Verification items for the finished model (mm, model axes). Face numbers are marked on the shaded views. A direction names the side the tool comes from. Coordinates: 2 decimals unless noted, no trailing zeros. Loops run counter-clockwise (first coordinate to the right, second up) from the corner with the lowest first, then second, coordinate; pieces in that order, holes last. Notation, with made-up numbers: (20, 76.25) -> (48, 76.25) arc R25 cw to (48, 97.25) -> close; hole circle Ø9 at (85, 81). An arc over 180 degrees is marked (long way). Answer as a JSON object with one key per item and string values. Group by question number.
Q1. Gauge pin test, flat ends, axial feed: pin 1 Ø1.6 at (y, z) = (-21, 1) entering from +X; pin 2 Ø2.5 at (y, z) = (-24.5, 1.5) entering from +X; pin 3 Ø1 at (x, z) = (13.5, 1) entering from -Y; pin 4 Ø5 at (y, z) = (10.5, -23.5) entering from +X. Record the tip position at first contact, or that the pin passes through.
Q2. Cross-section at D-D on x = 21. Record the boundary of the cut face in (y, z), and give its area (3 significant figures).
Q3. Set-up check for the marked faces 4, 5, 6 and 7: record each of +Z, -Z, +X, -X, +Y, -Y from which the full face is reachable in a straight line by a thin tool's end or side.
Q4. Cross-section at A-A on z = -20.5. Record the boundary of the cut face in (x, y), and give its area (3 significant figures).
Q5. Cross-section at C-C on y = -21. Record the boundary of the cut face in (x, z), and give its area (3 significant figures).
Q6. Cross-section at B-B on y = 16. Record the boundary of the cut face in (x, z), and give its area (3 significant figures).
Q7. Release check for a two-part mould opening along X. For the marked faces 1, 2 and 3 record: released by +X, released by -X, zero draft, split by the parting line, or undercut.
Q8. Scan lines: L1, parallel to Y at x = -41, z = -10.8; L2, parallel to X at y = 8, z = -29; L3, parallel to X at y = -16, z = 0.5. Record each from-to range of solid material in increasing order.
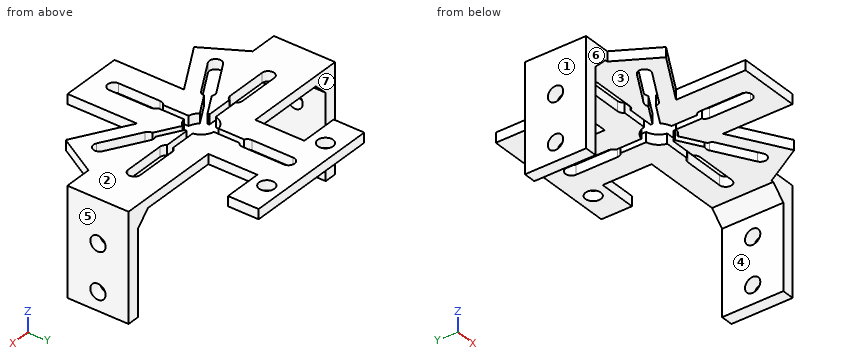
```python
from build123d import *

# Parameters (mm, degrees)
BOSS_EXTRUDE1_DEPTH = 3.2
SKETCH2_W           = 4
SKETCH2_H           = 20
BOSS_EXTRUDE2_DEPTH = 35
BOSS_EXTRUDE3_DEPTH = 20
CUT_EXTRUDE1_REACH  = 102.256
SKETCH4_R           = 2.5
SKETCH5_R           = 2.5
CUT_EXTRUDE2_DEPTH  = 3.2


with BuildPart() as part:
    # Sketch1 → Boss-Extrude1 (new body)
    with BuildSketch(Plane.XY):
        Polygon((22.5, 36), (-22.5, 36), (-22.5, 26), (-10, 26), (-10, 10), (-40, 10), (-40, -10), (-35, -10), (-27.320508076, -23.301270189), (-10, -13.301270189), (-10, -36), (10, -36), (10, -13.301270189), (27.320508076, -23.301270189), (35, -10), (40, -10), (40, 10), (10, 10), (10, 26), (22.5, 26), align=None)
        with BuildLine():
            Line((2, 28.5), (2, 15))
            ThreePointArc((2, 15), (1.732050808, 14), (1, 13.267949192))
            Line((1, 13.267949192), (1, 4.898979486))
            ThreePointArc((1, 4.898979486), (3.535533906, 3.535533906), (4.898979486, 1))
            Line((4.898979486, 1), (13.267949192, 1))
            ThreePointArc((13.267949192, 1), (14, 1.732050808), (15, 2))
            Line((15, 2), (28.5, 2))
            ThreePointArc((28.5, 2), (30.5, 0), (28.5, -2))
            Line((28.5, -2), (15, -2))
            ThreePointArc((15, -2), (14, -1.732050808), (13.267949192, -1))
            Line((13.267949192, -1), (4.898979486, -1))
            ThreePointArc((4.898979486, -1), (4.829629131, -1.294095226), (4.742640687, -1.583464339))
            Line((4.742640687, -1.583464339), (11.990381057, -5.767949192))
            ThreePointArc((11.990381057, -5.767949192), (12.990381057, -5.5), (13.990381057, -5.767949192))
            Line((13.990381057, -5.767949192), (25.681724008, -12.517949192))
            ThreePointArc((25.681724008, -12.517949192), (26.413774815, -15.25), (23.681724008, -15.982050808))
            Line((23.681724008, -15.982050808), (11.990381057, -9.232050808))
            ThreePointArc((11.990381057, -9.232050808), (11.258330249, -8.5), (10.990381057, -7.5))
            Line((10.990381057, -7.5), (3.742640687, -3.315515147))
            ThreePointArc((3.742640687, -3.315515147), (2.5, -4.330127019), (1, -4.898979486))
            Line((1, -4.898979486), (1, -13.267949192))
            ThreePointArc((1, -13.267949192), (1.732050808, -14), (2, -15))
            Line((2, -15), (2, -28.5))
            ThreePointArc((2, -28.5), (0, -30.5), (-2, -28.5))
            Line((-2, -28.5), (-2, -15))
            ThreePointArc((-2, -15), (-1.732050808, -14), (-1, -13.267949192))
            Line((-1, -13.267949192), (-1, -4.898979486))
            ThreePointArc((-1, -4.898979486), (-2.5, -4.330127019), (-3.742640687, -3.315515147))
            Line((-3.742640687, -3.315515147), (-10.990381057, -7.5))
            ThreePointArc((-10.990381057, -7.5), (-11.258330249, -8.5), (-11.990381057, -9.232050808))
            Line((-11.990381057, -9.232050808), (-23.681724008, -15.982050808))
            ThreePointArc((-23.681724008, -15.982050808), (-26.413774815, -15.25), (-25.681724008, -12.517949192))
            Line((-25.681724008, -12.517949192), (-13.990381057, -5.767949192))
            ThreePointArc((-13.990381057, -5.767949192), (-12.990381057, -5.5), (-11.990381057, -5.767949192))
            Line((-11.990381057, -5.767949192), (-4.742640687, -1.583464339))
            ThreePointArc((-4.742640687, -1.583464339), (-4.829629131, -1.294095226), (-4.898979486, -1))
            Line((-4.898979486, -1), (-13.267949192, -1))
            ThreePointArc((-13.267949192, -1), (-14, -1.732050808), (-15, -2))
            Line((-15, -2), (-28.5, -2))
            ThreePointArc((-28.5, -2), (-30.5, 0), (-28.5, 2))
            Line((-28.5, 2), (-15, 2))
            ThreePointArc((-15, 2), (-14, 1.732050808), (-13.267949192, 1))
            Line((-13.267949192, 1), (-4.898979486, 1))
            ThreePointArc((-4.898979486, 1), (-3.535533906, 3.535533906), (-1, 4.898979486))
            Line((-1, 4.898979486), (-1, 13.267949192))
            ThreePointArc((-1, 13.267949192), (-1.732050808, 14), (-2, 15))
            Line((-2, 15), (-2, 28.5))
            ThreePointArc((-2, 28.5), (0, 30.5), (2, 28.5))
        make_face(mode=Mode.SUBTRACT)
    extrude(amount=BOSS_EXTRUDE1_DEPTH)

    # Sketch2 → Boss-Extrude2 (add)
    with BuildSketch(Plane(origin=(0, 0, 3.2), x_dir=(-1, 0, 0), z_dir=(0, 0, -1))):
        with Locations((42, 0)):
            Rectangle(SKETCH2_W, SKETCH2_H)
        with Locations((-42, 0)):
            Rectangle(SKETCH2_W, SKETCH2_H)
    extrude(amount=BOSS_EXTRUDE2_DEPTH)

    # Sketch3 → Boss-Extrude3 (add)
    with BuildSketch(Plane(origin=(0, 10, 0), x_dir=(1, 0, 0), z_dir=(0, 1, 0))):
        Polygon((-40, 4.242640687), (-35.757359313, 0), (-40, 0), align=None)
        Polygon((35.757359313, 0), (40, 0), (40, 4.242640687), align=None)
    extrude(amount=-BOSS_EXTRUDE3_DEPTH)

    # Cut-Extrude1: up to this face of the body (flat: up to its plane)
    cut_extrude1_end = Plane(part.part.faces().sort_by_distance((44, 0, -14.3))[0])
    # Sketch4 → Cut-Extrude1 (cut, up to the picked face)
    with BuildSketch(Plane.ZY.offset(44), mode=Mode.PRIVATE) as cut_extrude1_sk1:
        with Locations((-25.8, 0)):
            Circle(SKETCH4_R)
    cut_extrude1_tool1 = split(extrude(cut_extrude1_sk1.sketch, amount=-CUT_EXTRUDE1_REACH, mode=Mode.PRIVATE), bisect_by=cut_extrude1_end, keep=Keep.BOTH, mode=Mode.PRIVATE)
    # Sketch4 → Cut-Extrude1 (cut, up to the picked face)
    with BuildSketch(Plane.ZY.offset(44), mode=Mode.PRIVATE) as cut_extrude1_sk2:
        with Locations((-10.8, 0)):
            Circle(SKETCH4_R)
    cut_extrude1_tool2 = split(extrude(cut_extrude1_sk2.sketch, amount=-CUT_EXTRUDE1_REACH, mode=Mode.PRIVATE), bisect_by=cut_extrude1_end, keep=Keep.BOTH, mode=Mode.PRIVATE)
    add(cut_extrude1_tool1.solids().sort_by(Axis((-44, 0, -25.8), (1, 0, 0)))[0], mode=Mode.SUBTRACT)
    add(cut_extrude1_tool2.solids().sort_by(Axis((-44, 0, -10.8), (1, 0, 0)))[0], mode=Mode.SUBTRACT)

    # Sketch5 → Cut-Extrude2 (cut)
    with BuildSketch(Plane.XY.offset(3.2)):
        with Locations((-12.5, 31)):
            Circle(SKETCH5_R)
        with Locations((12.5, 31)):
            Circle(SKETCH5_R)
    extrude(amount=-CUT_EXTRUDE2_DEPTH, mode=Mode.SUBTRACT)


solid = part.part
```
Computed values:
{
 "1": {"pin 1": "stops at x = 29.11", "pin 2": "stops at x = 27.35", "pin 3": "stops at y = -15.61", "pin 4": "stops at x = 44"},
 "2": {"outline": "(-19.65, 0) -> (-14.43, 0) -> (-14.43, 3.2) -> (-19.65, 3.2) -> close; (-9.81, 0) -> (-2, 0) -> (-2, 3.2) -> (-9.81, 3.2) -> close; (2, 0) -> (10, 0) -> (10, 3.2) -> (2, 3.2) -> close; (26, 0) -> (36, 0) -> (36, 3.2) -> (26, 3.2) -> close", "area": "99.3 mm²"},
 "3": {"face 4": "-Z, +Y, -Y", "face 5": "+Z, -Z, +X, +Y, -Y", "face 6": "+Z, -Z, -X, -Y", "face 7": "+Z, -Z, -X"},
 "4": {"outline": "(-44, -10) -> (-40, -10) -> (-40, 10) -> (-44, 10) -> close; (40, -10) -> (44, -10) -> (44, 10) -> (40, 10) -> close", "area": "160 mm²"},
 "5": {"outline": "(-28.65, 0) -> (-23.33, 0) -> (-23.33, 3.2) -> (-28.65, 3.2) -> close; (-10, 0) -> (-2, 0) -> (-2, 3.2) -> (-10, 3.2) -> close; (2, 0) -> (10, 0) -> (10, 3.2) -> (2, 3.2) -> close; (23.33, 0) -> (28.65, 0) -> (28.65, 3.2) -> (23.33, 3.2) -> close", "area": "85.2 mm²"},
 "6": {"outline": "(-10, 0) -> (-2, 0) -> (-2, 3.2) -> (-10, 3.2) -> close; (2, 0) -> (10, 0) -> (10, 3.2) -> (2, 3.2) -> close", "area": "51.2 mm²"},
 "7": {"face 1": "released by -X", "face 2": "zero draft", "face 3": "undercut"},
 "8": {"L1": "y = -10 to -2.5, 2.5 to 10", "L2": "x = -44 to -40, 40 to 44", "L3": "x = -31.54 to -25.65, -23.71 to -14.67, -10 to -2, 2 to 10, 14.67 to 23.71, 25.65 to 31.54"}
}
